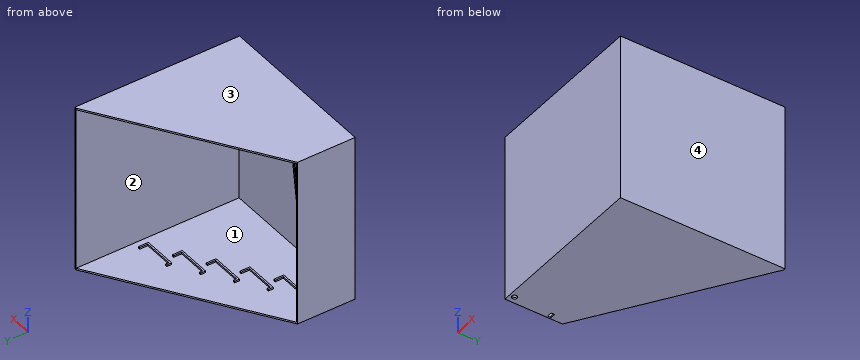
Autodesk Inventor part; units mm, degrees
ref_plane "Plano de trabalho1" through (0, 0, 500) normal (0, 0, 1) x (1, 0, 0)
ref_plane "YZ Plane" through (0, 0, 0) normal (1, 0, 0) x (0, 1, 0)
ref_plane "XZ Plane" through (0, 0, 0) normal (0, 1, 0) x (-1, 0, 0)
sketch "Esboço1" plane through (0, 0, 0) normal (0, 0, 1) x (1, 0, 0)
  line L0 (0, 0) -> (1000, 0)
  line L1 (1000, 0) -> (1000, 1000)
  line L2 (0, 0) -> (0, 350)
  line L3 (990, 1000) -> (990, 10)
  line L4 (990, 10) -> (10, 10)
  line L5 (10, 10) -> (10, 350)
  line L6 (0, 350) -> (10, 350)
  line L7 (990, 1000) -> (1000, 1000)
  line L8 (0, 350) -> (10, 350)
  line L9 (990, 1000) -> (1000, 1000)
  dimension "d6" = 1000
  dimension "d7" = 1000
  dimension "d8" = 350
  dimension "d10" = 10
extrude "Extrusão1" add sketch "Esboço1" along normal blind 1000
sketch "Esboço2" plane through (0, 0, 1000) normal (0, 0, 1) x (1, 0, 0)
  line L0 (10, 10) -> (10, 350)
  line L1 (0, 350) -> (0, 0)
  line L2 (1000, 1000) -> (990, 1000)
  line L3 (0, 350) -> (990, 1000)
  line L4 (0, 0) -> (1000, 0)
  line L5 (1000, 0) -> (1000, 1000)
  line L6 (0, 350) -> (0, 0)
  line L7 (1000, 0) -> (1000, 1000)
  line L8 (990, 1000) -> (1000, 1000)
extrude "Extrusão2" add sketch "Esboço2" along normal blind 10
sketch "Esboço3" plane through (0, 0, 0) normal (0, 0, -1) x (-1, 0, 0)
  line L0 (-10, 350) -> (0, 350)
  line L1 (-1000, 1000) -> (-990, 1000)
  line L2 (0, 350) -> (-990, 1000)
  line L3 (-990, 1000) -> (-1000, 1000)
  line L4 (-1000, 1000) -> (-1000, 0)
  line L5 (0, 0) -> (-1000, 0)
  line L6 (-1000, 0) -> (0, 0)
  line L7 (0, 0) -> (0, 350)
extrude "Extrusão3" add sketch "Esboço3" along normal blind 10
sketch "Esboço4" plane through (10, 10, 1000) normal (1, 0, 0) x (0, 0, -1)
  line L0 (1000, 990) -> (1000, 0)
  line L1 (1000, 232.5113) -> (0, 320)
  line L2 (0, 0) -> (0, 340)
  line L3 (0, 340) -> (-10, 340)
  line L4 (1000, 242.5495) -> (0, 330.0382)
  line L5 (1000, 232.5113) -> (1000, 242.5495)
  line L6 (1000, 0) -> (1000, 340)
  line L7 (0, 330.0382) -> (0, 320)
  point P0 (1000, -10)
  dimension "d11" = 85
  dimension "d13" = 20
  dimension "d14" = 10
extrude "Extrusão4" add sketch "Esboço4" along normal blind 30
sketch "Esboço5" plane through (40, 10, 1000) normal (1, 0, 0) x (0, 0, -1)
  line L0 (1000, 232.5113) -> (0, 320)
  line L1 (1000, 232.5113) -> (0, 320)
  line L2 (0, 336.0611) -> (1000, 248.5725)
  line L3 (1000, 242.5495) -> (1000, 340)
  line L4 (1000, 248.5725) -> (1000, 242.5495)
  line L5 (0, 336.0611) -> (0, 320)
  line L6 (0, 330.0382) -> (0, 340)
  line L7 (1000, 0) -> (1000, 232.5113)
  line L8 (1000, 232.5113) -> (0, 320)
  line L9 (0, 330.0382) -> (1000, 242.5495)
  point P0 (1000, -10)
  dimension "d18" = 6
extrude "Extrusão5" add sketch "Esboço5" along normal blind 10
sketch "Esboço6" plane through (0, 0, 0) normal (0, 0, 1) x (1, 0, 0)
  line L0 (10, 252.5495) -> (10, 350)
  line L1 (10, 252.5495) -> (40, 252.5495)
  line L2 (40, 252.5495) -> (40, 273.6954)
  line L3 (40, 273.6954) -> (10, 273.6954)
  line L4 (10, 273.6954) -> (10, 252.5495)
  point P0 (0, 0)
extrude "Extrusão6" cut sketch "Esboço6" against normal blind 10
sketch "Esboço7" plane through (0, 0, 0) normal (0, 0, 1) x (1, 0, 0)
  line L0 (0, 350) -> (990, 1000)
  line L1 (591.5971, 523.0033) -> (591.5971, 493.0033)
  line L2 (591.5971, 493.0033) -> (793.5971, 493.0033)
  line L3 (793.5971, 493.0033) -> (793.5971, 553.0033)
  line L4 (793.5971, 553.0033) -> (783.5971, 553.0033)
  line L5 (783.5971, 553.0033) -> (783.5971, 503.0033)
  line L6 (783.5971, 503.0033) -> (601.5971, 503.0033)
  line L7 (601.5971, 503.0033) -> (601.5971, 523.0033)
  line L8 (601.5971, 523.0033) -> (591.5971, 523.0033)
  line L9 (0, 0) -> (0, 350)
  line L10 (441.0647, 423.0033) -> (441.0647, 393.0033)
  line L11 (441.0647, 393.0033) -> (643.0647, 393.0033)
  line L12 (643.0647, 393.0033) -> (643.0647, 453.0033)
  line L13 (643.0647, 453.0033) -> (633.0647, 453.0033)
  line L14 (633.0647, 453.0033) -> (633.0647, 403.0033)
  line L15 (633.0647, 403.0033) -> (451.0647, 403.0033)
  line L16 (451.0647, 403.0033) -> (451.0647, 423.0033)
  line L17 (451.0647, 423.0033) -> (441.0647, 423.0033)
  line L18 (290.5324, 323.0033) -> (290.5324, 293.0033)
  line L19 (290.5324, 293.0033) -> (492.5324, 293.0033)
  line L20 (492.5324, 293.0033) -> (492.5324, 353.0033)
  line L21 (492.5324, 353.0033) -> (482.5324, 353.0033)
  line L22 (482.5324, 353.0033) -> (482.5324, 303.0033)
  line L23 (482.5324, 303.0033) -> (300.5324, 303.0033)
  line L24 (300.5324, 303.0033) -> (300.5324, 323.0033)
  line L25 (300.5324, 323.0033) -> (290.5324, 323.0033)
  line L26 (140, 223.0033) -> (140, 193.0033)
  line L27 (140, 193.0033) -> (342, 193.0033)
  line L28 (342, 193.0033) -> (342, 253.0033)
  line L29 (342, 253.0033) -> (332, 253.0033)
  line L30 (332, 253.0033) -> (332, 203.0033)
  line L31 (332, 203.0033) -> (150, 203.0033)
  line L32 (150, 203.0033) -> (150, 223.0033)
  line L33 (150, 223.0033) -> (140, 223.0033)
  line L34 (0, 100) -> (1000, 764.309)
  line L35 (1000, 1000) -> (1000, 0)
  line L36 (742.1294, 623.0033) -> (742.1294, 593.0033)
  line L37 (742.1294, 593.0033) -> (944.1294, 593.0033)
  line L38 (944.1294, 593.0033) -> (944.1294, 653.0033)
  line L39 (944.1294, 653.0033) -> (934.1294, 653.0033)
  line L40 (934.1294, 653.0033) -> (934.1294, 603.0033)
  line L41 (934.1294, 603.0033) -> (752.1294, 603.0033)
  line L42 (752.1294, 603.0033) -> (752.1294, 623.0033)
  line L43 (752.1294, 623.0033) -> (742.1294, 623.0033)
  dimension "d23" = 202
  dimension "d24" = 10
  dimension "d25" = 10
  dimension "d26" = 10
  dimension "d27" = 30
  dimension "d28" = 60
  dimension "d35" = 202
  dimension "d36" = 10
  dimension "d37" = 10
  dimension "d38" = 10
  dimension "d39" = 30
  dimension "d40" = 60
  dimension "d41" = 202
  dimension "d42" = 10
  dimension "d43" = 10
  dimension "d44" = 10
  dimension "d45" = 30
  dimension "d46" = 60
  dimension "d47" = 202
  dimension "d48" = 10
  dimension "d49" = 10
  dimension "d50" = 10
  dimension "d51" = 30
  dimension "d52" = 60
  dimension "d53" = 100
  dimension "d54" = 202
  dimension "d55" = 10
  dimension "d56" = 10
  dimension "d57" = 10
  dimension "d58" = 30
  dimension "d59" = 60
  dimension "d60" = 90
  dimension "d61" = 90
  dimension "d62" = 90
  dimension "d63" = 90
  dimension "d64" = 764.309
  dimension "d65" = 140
extrude "Extrusão7" add sketch "Esboço7" along normal blind 10
ref_plane "Plano de trabalho1" through (0, 0, 500) normal (0, 0, 1) x (1, 0, 0)
mirror "Espelhamento1" about plane through (0, 0, 500) normal (0, 0, 1) of "Extrusão7"
sketch "Esboço8" plane through (0, 0, 0) normal (0, 0, 1) x (1, 0, 0)
  circle A0 centre (41.0461, 30) radius 15.525
  line L0 (990, 10) -> (10, 10)
  point P0 (0, 0)
  dimension "d68" = 31.05
  dimension "d69" = 20
extrude "Extrusão8" cut sketch "Esboço8" against normal blind 10
properties part number "caixa" material "Polipropileno"
CAD build for the part. Positions are in the model's coordinates, mm. Face numbers are marked on the shaded views. Give positions to 0.01 mm unless a question says otherwise; leave off trailing zeros. Write each loop counter-clockwise with the first axis right and the second up, starting at its lowest first coordinate (ties: lowest second). Pieces come first, ordered by that corner, then holes. Notation, with made-up numbers: M -0.5,78 L 54.5,78 A19 ccw 54.5,113 Z; hole C 73.25,71.25 d9. An arc over 180 degrees is marked long. Put each result on its own line as item: value. Start each with the question number.
(1) Mould opens along X. For the marked faces 1, 2, 3 and 4 say: +X half, -X half, draft (parallel to the pull), parting line (faces both ways), or undercut.
(2) Flat gauge pins, fed straight in: pin 1 Ø3 at (x, z) = (405.5, 418.5) entering from -Y; pin 2 Ø25 at (x, y) = (41.05, 30) entering from -Z; pin 3 Ø5 at (y, z) = (435.5, 994) entering from -X; pin 4 Ø1 at (x, z) = (802, 867.5) entering from +Y. Where does each tip first touch, or does it go through?
(3) Band-saw the part on C-C, the plane x = 178. Write the cut outline in (y, z), and give its area (3 significant figures).
(4) Probe L1, parallel to Z at x = 756, y = 725.5; L2, parallel to Z at x = 437, y = 293.5; L3, parallel to X at y = 179.5, z = 304. List the from-to ranges inside material, lowest first.
(5) Band-saw the part on A-A, the plane y = 30. Write the cut outline in (x, z).
Response values:
1. face 1: undercut
1. face 2: undercut
1. face 3: draft
1. face 4: +X half
2. pin 1: stops at y = 0
2. pin 2: stops at z = 1000
2. pin 3: stops at x = 633.06
2. pin 4: stops at y = 10
3. outline: M 0,-10 L 466.87,-10 L 466.87,0 L 203,0 L 203,10 L 193,10 L 193,0 L 10,0 L 10,1000 L 193,1000 L 193,990 L 203,990 L 203,1000 L 466.87,1000 L 466.87,1010 L 0,1010 Z
3. area: 19,500 mm2
4. L1: z = -10 to 0, 1000 to 1010
4. L2: z = -10 to 10, 990 to 1010
4. L3: x = 0 to 10, 990 to 1000
5. outline: M 0,-10 L 25.52,-10 L 25.52,0 L 10,0 L 10,1000 L 990,1000 L 990,0 L 56.57,0 L 56.57,-10 L 1000,-10 L 1000,1010 L 0,1010 Z
